Autodesk Inventor part; units mm, degrees
ref_plane "Work Plane1" through (0, 0.2202, 0) normal (0, 0, 1) x (1, 0, 0)
ref_plane "YZ Plane" through (0, 0, 0) normal (1, 0, 0) x (0, 1, 0)
ref_plane "XZ Plane" through (0, 0, 0) normal (0, 1, 0) x (-1, 0, 0)
ref_plane "Work Plane1" through (0, 0.2202, 0) normal (0, 0, 1) x (1, 0, 0)
sketch "Sketch1" plane through (0, 0.2202, 0) normal (0, 0, 1) x (1, 0, 0)
  line L0 (21.9247, 42.5927) -> (36.4247, 42.5927)
  line L1 (36.4247, 42.5927) -> (36.4247, 36.8927)
  line L2 (36.4247, 36.8927) -> (21.9247, 36.8927)
  line L3 (21.9247, 36.8927) -> (21.9247, 42.5927)
  point P0 (0, -0.2202)
  dimension "d0" = 14.5
  dimension "d2" = 5.7
extrude "Extrusion1" add sketch "Sketch1" along normal blind 13.2
sketch "Sketch2" plane through (36.4247, 37.1129, 0) normal (1, 0, 0) x (0, 0, -1)
  line L0 (0, 5.7) -> (0, 0)
  line L1 (0, 5.7) -> (-13.2, 5.7)
  line L2 (-13.2, 0) -> (-13.2, 5.7)
  line L3 (0, 0) -> (-13.2, 0)
  line L4 (-12.8, 5.3) -> (-0.4, 5.3)
  line L5 (-0.4, 5.3) -> (-0.4, 0.4)
  line L6 (-0.4, 0.4) -> (-12.8, 0.4)
  line L7 (-12.8, 0.4) -> (-12.8, 5.3)
  point P0 (0, -37.1129)
  dimension "d5" = 0.4
extrude "Extrusion2" cut sketch "Sketch2" against normal blind 13 contours L4 L5 L6 L7
sketch "Sketch3" plane through (23.4247, 37.1129, 0) normal (1, 0, 0) x (0, 0, -1)
  line L0 (-12.8, 0.4) -> (-12.8, 5.3)
  line L1 (-0.4, 0.4) -> (-12.8, 0.4)
  line L2 (-0.4, 5.3) -> (-0.4, 0.4)
  line L3 (-12.6, 2) -> (-0.6, 2)
  line L4 (-0.6, 2) -> (-0.6, 0.6)
  line L5 (-0.6, 0.6) -> (-12.6, 0.6)
  line L6 (-12.6, 0.6) -> (-12.6, 2)
  point P0 (0, -37.1129)
  dimension "d8" = 0.2
  dimension "d9" = 0.2
  dimension "d10" = 0.2
  dimension "d11" = 1.4
extrude "Extrusion3" add sketch "Sketch3" along normal blind 13
pattern_linear "Rectangular Pattern1" count 2 spacing 5.5 along (0, 1, 0) of "Extrusion1", "Extrusion3", "Extrusion2"
properties part number "nanopc_t4_usb"
Design review of the part built by this model. Coordinates are the model's own, in mm. A direction names the side the tool comes from. Round coordinates to 2 decimals unless told otherwise and drop trailing zeros. Loops run counter-clockwise (first coordinate to the right, second up) from the corner with the lowest first, then second, coordinate; pieces in that order, holes last. Notation, with made-up numbers: M -0.5,-14.75 L 49.5,-14.75 A11 cw 49.5,-9.75 Z; hole C -24.5,66 d11. An arc over 180 degrees is marked long. Answer as a JSON object with one key per item and string values.
Item 1: We need section D-D on y = 47.5. Give the boundary of the cut face in (x, z), and give its area (3 significant figures).
Answer sheet:
{"outline": "M 21.92,0 L 36.42,0 L 36.42,0.4 L 23.42,0.4 L 23.42,12.8 L 36.42,12.8 L 36.42,13.2 L 21.92,13.2 Z", "area": "30.2 mm^2"}
Item 2: We need section B-B on y = 43.5. Give the boundary of the cut face in (x, z).
Answer sheet:
{"outline": "M 21.92,0 L 36.42,0 L 36.42,0.4 L 23.42,0.4 L 23.42,0.6 L 36.42,0.6 L 36.42,12.6 L 23.42,12.6 L 23.42,12.8 L 36.42,12.8 L 36.42,13.2 L 21.92,13.2 Z"}
Item 3: The part is to be moulded in two halves that separate along Z. For faces 1 (the flat face through (36.425, 38, 7)), 2 (the flat face through (30, 45, 0.4)), 3 (the flat face through (29, 43, 0)), say which applies: pulls with the +Z half, pulls with the -Z half, needs draft (parallel to the pull), parting line crosses it, or undercut.
Answer sheet:
{"face 1": "needs draft", "face 2": "undercut", "face 3": "pulls with the -Z half"}
Item 4: Machinability: for faces 4 (the flat face through (30, 42.413, 7)), 5 (the flat face through (36.425, 42.7, 6.6)), which of the approach directions +Z, -Z, +X, -X, +Y, -Y give a long, thin tool a straight path to every point of the face, cutting with its end or side? Answer none if there is none.
Answer sheet:
{"face 4": "+X", "face 5": "+Z, -Z, +X, +Y, -Y"}
Item 5: Clearance check with a flat-ended pin moving along its axis: P1, Ø4, axis at x = 31, y = 44, coming from the -Z side. State where the tip first meets the part, or that it passes through.
Answer sheet:
{"P1": "stops at z = 0"}
Item 6: Wall thickness on L1, parallel to Y at x = 29.5, z = 2; L2, parallel to Z at x = 32.25, y = 38; L3, parallel to Z at x = 29.5, y = 42.25: over which ranges is each line inside the solid? List them lowest first. Write a range as from..to.
Answer sheet:
{"L1": "y = 37.11..37.51, 37.71..39.11, 42.41..43.01, 43.21..44.61, 47.91..48.31", "L2": "z = 0..0.4, 0.6..12.6, 12.8..13.2", "L3": "z = 0..0.4, 12.8..13.2"}
Item 7: We need section C-C on z = 6.25. Give the boundary of the cut face in (x, y), and give its area (3 significant figures).
Answer sheet:
{"outline": "M 21.92,37.11 L 36.42,37.11 L 36.42,37.51 L 23.42,37.51 L 23.42,37.71 L 36.42,37.71 L 36.42,39.11 L 23.42,39.11 L 23.42,42.41 L 36.42,42.41 L 36.42,43.01 L 23.42,43.01 L 23.42,43.21 L 36.42,43.21 L 36.42,44.61 L 23.42,44.61 L 23.42,47.91 L 36.42,47.91 L 36.42,48.31 L 21.92,48.31 Z", "area": "71.4 mm^2"}
Item 8: We need section A-A on x = 25.5. Give the boundary of the cut face in (y, z), and give its area (3 significant figures).
Answer sheet:
{"outline": "M 37.11,0 L 48.31,0 L 48.31,13.2 L 37.11,13.2 Z; M 37.71,0.6 L 39.11,0.6 L 39.11,12.6 L 37.71,12.6 Z; M 43.21,0.6 L 44.61,0.6 L 44.61,12.6 L 43.21,12.6 Z; hole M 37.51,0.4 L 42.41,0.4 L 42.41,12.8 L 37.51,12.8 Z; hole M 43.01,0.4 L 47.91,0.4 L 47.91,12.8 L 43.01,12.8 Z", "area": "59.9 mm^2"}
